Job drawing, mm, ordinate dimensions from the low corner. One solid piece. Give positions to 0.01 mm unless a question says otherwise; leave off trailing zeros. Write each loop counter-clockwise with the first axis right and the second up, starting at its lowest first coordinate (ties: lowest second). Pieces come first, ordered by that corner, then holes. Notation, with made-up numbers: M 21,-26.75 L 38,-26.75 A20 ccw 38,10.25 Z; hole C 54,14.25 d9. An arc over 180 degrees is marked long. Answer as CSV lines item,"result". Start each with the question number.
1) Slice it at A-A, the plane z = 3.25. Give the cut face in (x, y).
2) Wall check: line 1 along Y through (x, z) = (2.25, 3.25); line 2 along Y through (x, z) = (0.5, 3.5); line 3 along Z through (x, y) = (5, 4). Give the ranges that are in metal, low to high. Write a range as from..to.
3) Slice it at C-C, the plane y = 16. Give the cut face in (x, z), plus the area to 3 significant figures.
4) Mould opens along Y. For the marked faces 1 and 2 say: pulls with the +Y half, pulls with the -Y half, needs draft (parallel to the pull), parting line crosses it, or undercut.
5) Slice it at B-B, the plane y = 4. Give the cut face in (x, z).
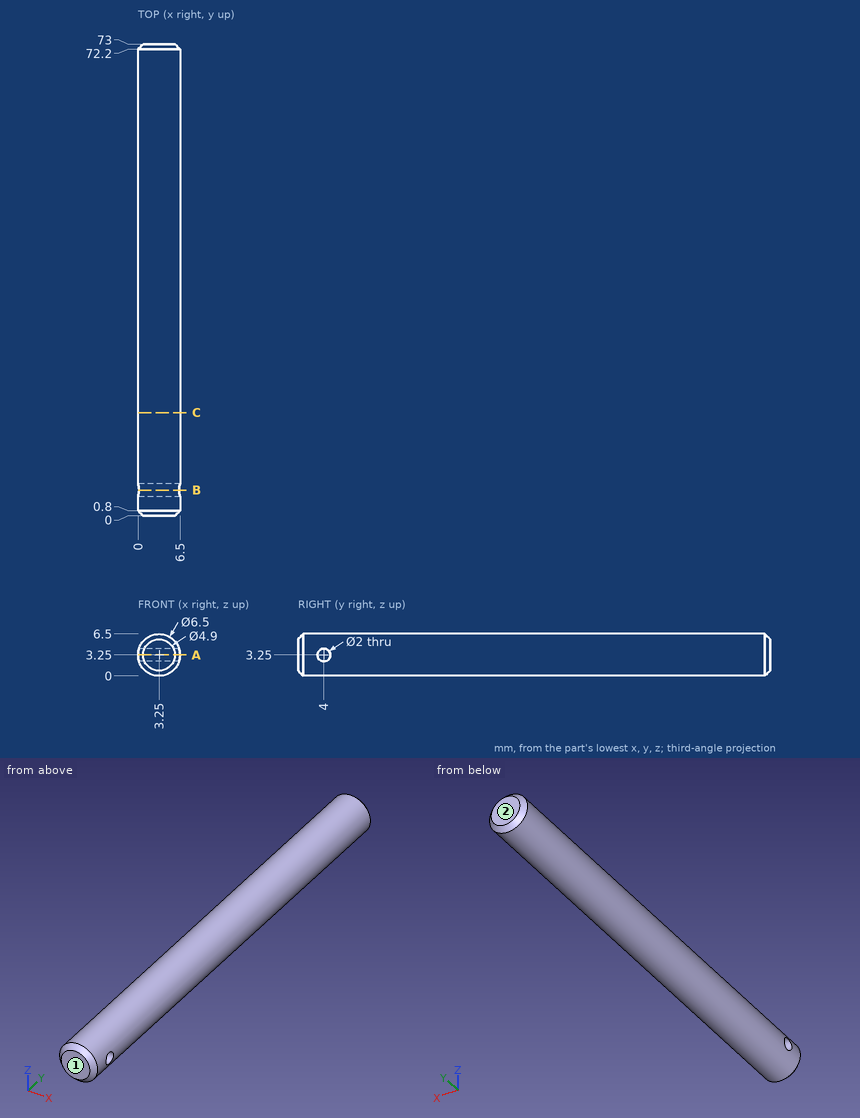
Found:
1,outline,"M 0,0.8 L 0.8,0 L 5.7,0 L 6.5,0.8 L 6.5,3 L 0,3 Z; M 0,5 L 6.5,5 L 6.5,72.2 L 5.7,73 L 0.8,73 L 0,72.2 Z"
2,line 1,"0..3, 5..73"
2,line 2,"0.31..3.03, 4.97..72.69"
2,line 3,"0.51..2.25, 4.25..5.99"
3,outline,"C 3.25,3.25 d6.5"
3,area,"33.2 mm²"
4,face 1,"pulls with the -Y half"
4,face 2,"pulls with the +Y half"
5,outline,"M 0.16,2.25 A3.25 ccw 6.34,2.25 Z; M 0.16,4.25 L 6.34,4.25 A3.25 ccw Z"
